Part model, mm, in its own coordinate system. A direction names the side the tool comes from. Give positions to 0.01 mm unless a question says otherwise; leave off trailing zeros. Write each loop counter-clockwise with the first axis right and the second up, starting at its lowest first coordinate (ties: lowest second). Pieces come first, ordered by that corner, then holes.
from build123d import *

# Parameters (mm, degrees)
SKETCH1_W               = 62
SKETCH1_H               = 48
BOSS_EXTRUDE1_DEPTH     = 5
SKETCH2_R               = 1.65
CUT_EXTRUDE2_DEPTH      = 5
SKETCH3_R               = 11
SKETCH3_R_2             = 1.65
BOSS_EXTRUDE2_DEPTH     = 2
SKETCH4_R               = 9.6
CUT_EXTRUDE4_DEPTH      = 5
SKETCH5_W               = 5
SKETCH5_H               = 35
BOSS_EXTRUDE3_DEPTH     = 25
CUT_EXTRUDE5_DEPTH      = 60.860253925
CUT_EXTRUDE5_DEPTH_BACK = 25
SKETCH6_R               = 1.15
SKETCH7_R               = 1.65
CUT_EXTRUDE6_DEPTH      = 5
SKETCH8_R               = 11
CUT_EXTRUDE7_DEPTH      = 65.536811201
SKETCH9_W               = 19
SKETCH9_H               = 60
BOSS_EXTRUDE4_DEPTH     = 3
SKETCH10_W              = 19
SKETCH10_H              = 55
BOSS_EXTRUDE5_DEPTH     = 3.7
SKETCH11_W              = 5
SKETCH11_H              = 48
BOSS_EXTRUDE6_DEPTH     = 25
BOSS_EXTRUDE7_DEPTH     = 3.7
SKETCH13_R              = 31
SKETCH13_R_2            = 28.5
BOSS_EXTRUDE8_DEPTH     = 25
SKETCH14_W              = 62
SKETCH14_H              = 5
BOSS_EXTRUDE9_DEPTH     = 10
SKETCH15_R              = 8
SKETCH15_R_2            = 7
BOSS_EXTRUDE10_DEPTH    = 7
CHAMFER1_SIZE           = 5
CUT_EXTRUDE8_DEPTH      = 109.894444303
CUT_EXTRUDE8_DEPTH_BACK = 109.894444303
SKETCH16_R              = 0.9
CHAMFER2_SIZE           = 5
SKETCH17_W              = 19
SKETCH17_H              = 60
CUT_EXTRUDE9_DEPTH      = 10
SKETCH18_W              = 30
SKETCH18_H              = 44.3
CUT_EXTRUDE10_DEPTH     = 10
CHAMFER3_SIZE           = 5


with BuildPart() as part:
    # Sketch1 → Boss-Extrude1 (new body)
    with BuildSketch(Plane.XY):
        Rectangle(SKETCH1_W, SKETCH1_H)
    extrude(amount=BOSS_EXTRUDE1_DEPTH)

    # Sketch2 → Cut-Extrude2 (cut)
    with BuildSketch(Plane.XY.offset(5)):
        with Locations((6, 7)):
            Circle(SKETCH2_R)
        with Locations((13, 0)):
            Circle(SKETCH2_R)
        with Locations((6, -7)):
            Circle(SKETCH2_R)
        with Locations((-1, 0)):
            Circle(SKETCH2_R)
    extrude(amount=-CUT_EXTRUDE2_DEPTH, mode=Mode.SUBTRACT)

    # Sketch3 → Boss-Extrude2 (add)
    with BuildSketch(Plane(origin=(0, 0, 0), x_dir=(-1, 0, 0), z_dir=(0, 0, -1))):
        with Locations(Location((-6, 0, 0), (0, 0, 180))):
            Circle(SKETCH3_R)
        with Locations(Location((1, 0, 0), (0, 0, 180))):
            Circle(SKETCH3_R_2, mode=Mode.SUBTRACT)
        with Locations(Location((-6, -7, 0), (0, 0, 180))):
            Circle(SKETCH3_R_2, mode=Mode.SUBTRACT)
        with Locations(Location((-13, 0, 0), (0, 0, 180))):
            Circle(SKETCH3_R_2, mode=Mode.SUBTRACT)
        with Locations(Location((-6, 7, 0), (0, 0, 180))):
            Circle(SKETCH3_R_2, mode=Mode.SUBTRACT)
    extrude(amount=BOSS_EXTRUDE2_DEPTH)

    # Sketch4 → Cut-Extrude4 (cut)
    with BuildSketch(Plane.XY.offset(5)):
        with Locations((6, 0)):
            Circle(SKETCH4_R)
    extrude(amount=-CUT_EXTRUDE4_DEPTH, mode=Mode.SUBTRACT)

    # Sketch5 → Boss-Extrude3 (add)
    with BuildSketch(Plane.XY.offset(5)):
        Polygon((8.15, -17.5), (8.15, -24), (31, -24), (31, -17.5), (26, -17.5), align=None)
        with Locations((28.5, 0)):
            Rectangle(SKETCH5_W, SKETCH5_H)
        Polygon((8.15, 17.5), (26, 17.5), (31, 17.5), (31, 24), (8.15, 24), align=None)
    extrude(amount=BOSS_EXTRUDE3_DEPTH)

    # Sketch6 → Cut-Extrude5 (cut, two sides: drawn at the far end of the back side and taken through both)
    with BuildSketch(Plane(origin=(0, -17.5, 0), x_dir=(1, 0, 0), z_dir=(0, 1, 0)).offset(-CUT_EXTRUDE5_DEPTH_BACK)):
        with Locations((20, -27.75)):
            Circle(SKETCH6_R)
        with Locations((20, -7.25)):
            Circle(SKETCH6_R)
        with Locations((-0.7, -7.25)):
            Circle(SKETCH6_R)
        with Locations((-0.7, -27.75)):
            Circle(SKETCH6_R)
    extrude(amount=CUT_EXTRUDE5_DEPTH + CUT_EXTRUDE5_DEPTH_BACK, mode=Mode.SUBTRACT)

    # Sketch7 → Cut-Extrude6 (cut)
    with BuildSketch(Plane(origin=(0, 24, 0), x_dir=(1, 0, 0), z_dir=(0, 1, 0))):
        with Locations((0.45, -7.25)):
            Circle(SKETCH7_R)
        with Locations(Location((20, -7.25, 0), (0, 0, 270))):
            Circle(SKETCH7_R)
        with Locations(Location((20, -27.75, 0), (0, 0, 270))):
            Circle(SKETCH7_R)
        with Locations((0.45, -27.75)):
            Circle(SKETCH7_R)
    cut_extrude6 = extrude(amount=-CUT_EXTRUDE6_DEPTH, mode=Mode.SUBTRACT)

    # Mirror1: Cut-Extrude6 across plane
    add(cut_extrude6.mirror(Plane.ZX), mode=Mode.SUBTRACT)

    # Sketch8 → Cut-Extrude7 (cut, through all)
    with BuildSketch(Plane(origin=(0, 24, 0), x_dir=(1, 0, 0), z_dir=(0, 1, 0))):
        with Locations((1.65, -17.5)):
            Circle(SKETCH8_R)
    extrude(amount=-CUT_EXTRUDE7_DEPTH, mode=Mode.SUBTRACT)

    # Sketch9 → Boss-Extrude4 (add)
    with BuildSketch(Plane(origin=(0, 24, 0), x_dir=(1, 0, 0), z_dir=(0, 1, 0))):
        with Locations((17.65, -60)):
            Rectangle(SKETCH9_W, SKETCH9_H)
    extrude(amount=-BOSS_EXTRUDE4_DEPTH)

    # Sketch10 → Boss-Extrude5 (add)
    with BuildSketch(Plane(origin=(0, 24, 0), x_dir=(1, 0, 0), z_dir=(0, 1, 0))):
        with Locations((17.65, -62.5)):
            Rectangle(SKETCH10_W, SKETCH10_H)
    extrude(amount=BOSS_EXTRUDE5_DEPTH)

    # Sketch11 → Boss-Extrude6 (add)
    with BuildSketch(Plane.XY.offset(5)):
        with Locations((-28.5, 0)):
            Rectangle(SKETCH11_W, SKETCH11_H)
    extrude(amount=BOSS_EXTRUDE6_DEPTH)

    # Sketch12 → Boss-Extrude7 (add)
    with BuildSketch(Plane.XZ.offset(24)):
        with BuildLine():
            Line((-31, 30), (31, 30))
            Line((31, 30), (31, 65))
            ThreePointArc((31, 65), (0, 96), (-31, 65))
            Line((-31, 65), (-31, 30))
        make_face()
    extrude(amount=-BOSS_EXTRUDE7_DEPTH)

    # Sketch13 → Boss-Extrude8 (add)
    with BuildSketch(Plane(origin=(0, -20.3, 0), x_dir=(1, 0, 0), z_dir=(0, 1, 0))):
        with Locations((0, -65)):
            Circle(SKETCH13_R)
        with Locations(Location((0, -65, 0), (0, 0, 270))):
            Circle(SKETCH13_R_2, mode=Mode.SUBTRACT)
    extrude(amount=BOSS_EXTRUDE8_DEPTH)

    # Sketch14 → Boss-Extrude9 (add)
    with BuildSketch(Plane(origin=(0, 24, 0), x_dir=(1, 0, 0), z_dir=(0, 1, 0))):
        with Locations((0, -2.5)):
            Rectangle(SKETCH14_W, SKETCH14_H)
    extrude(amount=BOSS_EXTRUDE9_DEPTH)

    # Sketch15 → Boss-Extrude10 (add)
    with BuildSketch(Plane(origin=(0, 34, 0), x_dir=(1, 0, 0), z_dir=(0, 1, 0))):
        with Locations(Location((0, -2.5, 0), (0, 0, 18.209956864))):
            Circle(SKETCH15_R)
        with Locations(Location((0, -2.5, 0), (0, 0, 159.075167572))):
            Circle(SKETCH15_R_2, mode=Mode.SUBTRACT)
    extrude(amount=BOSS_EXTRUDE10_DEPTH)

    # Chamfer1
    # the kernel refuses this chamfer: 5 mm, written as the material it adds along each edge
    with BuildSketch(Plane(origin=(0, 34, 2.5), x_dir=(0.34706049300703296, 0, -0.9378427449171398), z_dir=(0.9378427449171398, 0, 0.34706049300703296))) as chamfer1_piece_1_section:
        Polygon((8 + CHAMFER1_SIZE, 0), (8, CHAMFER1_SIZE), (8, 0), align=None)
    chamfer1_piece_1 = revolve(axis=Axis((0, 34, 2.5), (0, 1, 0)), revolution_arc=220.61525354, mode=Mode.PRIVATE)
    chamfer1_piece_1 = split(chamfer1_piece_1, bisect_by=Plane(origin=(-9.551791351, 35.668281916, 5), z_dir=(0, 0, -1)), keep=Keep.TOP, mode=Mode.PRIVATE)
    chamfer1_piece_1 = split(chamfer1_piece_1, bisect_by=Plane(origin=(-9.551791351, 35.668281916, 0), z_dir=(0, 0, 1)), keep=Keep.TOP, mode=Mode.PRIVATE)
    add(chamfer1_piece_1)
    with BuildSketch(Plane(origin=(0, 34, 2.5), x_dir=(-0.3470604930069759, 0, 0.9378427449171609), z_dir=(-0.9378427449171609, 0, -0.3470604930069759))) as chamfer1_piece_2_section:
        Polygon((8 + CHAMFER1_SIZE, 0), (8, CHAMFER1_SIZE), (8, 0), align=None)
    chamfer1_piece_2 = revolve(axis=Axis((0, 34, 2.5), (0, 1, 0)), revolution_arc=220.61525354, mode=Mode.PRIVATE)
    chamfer1_piece_2 = split(chamfer1_piece_2, bisect_by=Plane(origin=(9.551791351, 35.668281916, 5), z_dir=(0, 0, -1)), keep=Keep.TOP, mode=Mode.PRIVATE)
    chamfer1_piece_2 = split(chamfer1_piece_2, bisect_by=Plane(origin=(9.551791351, 35.668281916, 0), z_dir=(0, 0, 1)), keep=Keep.TOP, mode=Mode.PRIVATE)
    add(chamfer1_piece_2)

    # Sketch16 → Cut-Extrude8 (cut, two sides: drawn at the far end of the back side and taken through both)
    with BuildSketch(Plane(origin=(0, 0, 0), x_dir=(-1, 0, 0), z_dir=(0, 0, -1)).offset(-CUT_EXTRUDE8_DEPTH_BACK)):
        with Locations((0, 37.406113714)):
            Circle(SKETCH16_R)
    extrude(amount=CUT_EXTRUDE8_DEPTH + CUT_EXTRUDE8_DEPTH_BACK, mode=Mode.SUBTRACT)

    # Chamfer2
    # the kernel refuses this chamfer: 5 mm, written as the material it adds along each edge
    with BuildSketch(Plane(origin=(6.320066525, 34, 5), x_dir=(0, -0.9996219169112968, -0.027495876610586317), z_dir=(-1, 0, 0))) as chamfer2_piece_1_section:
        Polygon((CHAMFER2_SIZE * 0.999621916911, CHAMFER2_SIZE * 0.0274958766106), (-CHAMFER2_SIZE * 0.0274958766106, CHAMFER2_SIZE * 0.999621916911), (0, 0), align=None)
    chamfer2_piece_1 = extrude(amount=26.777823541, mode=Mode.PRIVATE)
    chamfer2_piece_1 = chamfer2_piece_1 & Plane(origin=(0, 31.52085101, 2.5), x_dir=(0.94991775959971, 0, -0.31249999999530786), z_dir=(0, -1, 0)) * Cylinder(8, 74, mode=Mode.PRIVATE)
    chamfer2_piece_1 = chamfer2_piece_1 - Plane(origin=(0, 31.52085101, 2.5), x_dir=(-0.9340497736136041, 0, -0.3571428571487537), z_dir=(0, -1, 0)) * Cylinder(7, 74, mode=Mode.PRIVATE)
    add(chamfer2_piece_1)
    with BuildSketch(Plane(origin=(20.457757017, 34, 5), x_dir=(0, -0.9996219169112968, -0.027495876610586317), z_dir=(-1, 0, 0))) as chamfer2_piece_2_section:
        Polygon((CHAMFER2_SIZE * 0.999621916911, CHAMFER2_SIZE * 0.0274958766106), (-CHAMFER2_SIZE * 0.0274958766106, CHAMFER2_SIZE * 0.999621916911), (0, 0), align=None)
    chamfer2_piece_2 = extrude(amount=26.777823541, mode=Mode.PRIVATE)
    chamfer2_piece_2 = chamfer2_piece_2 & Plane(origin=(0, 31.52085101, 2.5), x_dir=(0.94991775959971, 0, -0.31249999999530786), z_dir=(0, -1, 0)) * Cylinder(8, 74, mode=Mode.PRIVATE)
    chamfer2_piece_2 = chamfer2_piece_2 - Plane(origin=(0, 31.52085101, 2.5), x_dir=(-0.9340497736136041, 0, -0.3571428571487537), z_dir=(0, -1, 0)) * Cylinder(7, 74, mode=Mode.PRIVATE)
    add(chamfer2_piece_2)
    with BuildSketch(Plane(origin=(-6.320066525, 34, 0), x_dir=(0, -0.9996219169112968, 0.027495876610586372), z_dir=(1, 0, 0))) as chamfer2_piece_3_section:
        Polygon((CHAMFER2_SIZE * 0.999621916911, CHAMFER2_SIZE * 0.0274958766106), (-CHAMFER2_SIZE * 0.0274958766106, CHAMFER2_SIZE * 0.999621916911), (0, 0), align=None)
    chamfer2_piece_3 = extrude(amount=26.777823541, mode=Mode.PRIVATE)
    chamfer2_piece_3 = chamfer2_piece_3 & Plane(origin=(0, 31.52085101, 2.5), x_dir=(0.94991775959971, 0, -0.31249999999530786), z_dir=(0, -1, 0)) * Cylinder(8, 74, mode=Mode.PRIVATE)
    chamfer2_piece_3 = chamfer2_piece_3 - Plane(origin=(0, 31.52085101, 2.5), x_dir=(-0.9340497736136041, 0, -0.3571428571487537), z_dir=(0, -1, 0)) * Cylinder(7, 74, mode=Mode.PRIVATE)
    add(chamfer2_piece_3)
    with BuildSketch(Plane(origin=(-20.457757017, 34, 0), x_dir=(0, -0.9996219169112968, 0.027495876610586372), z_dir=(1, 0, 0))) as chamfer2_piece_4_section:
        Polygon((CHAMFER2_SIZE * 0.999621916911, CHAMFER2_SIZE * 0.0274958766106), (-CHAMFER2_SIZE * 0.0274958766106, CHAMFER2_SIZE * 0.999621916911), (0, 0), align=None)
    chamfer2_piece_4 = extrude(amount=26.777823541, mode=Mode.PRIVATE)
    chamfer2_piece_4 = chamfer2_piece_4 & Plane(origin=(0, 31.52085101, 2.5), x_dir=(0.94991775959971, 0, -0.31249999999530786), z_dir=(0, -1, 0)) * Cylinder(8, 74, mode=Mode.PRIVATE)
    chamfer2_piece_4 = chamfer2_piece_4 - Plane(origin=(0, 31.52085101, 2.5), x_dir=(-0.9340497736136041, 0, -0.3571428571487537), z_dir=(0, -1, 0)) * Cylinder(7, 74, mode=Mode.PRIVATE)
    add(chamfer2_piece_4)
    with BuildSketch(Plane(origin=(-31, -20.3, 30), x_dir=(0, -0.027495876610586317, 0.9996219169112968), z_dir=(1, 0, 0))) as chamfer2_piece_5:
        Polygon((CHAMFER2_SIZE * 0.999621916911, -CHAMFER2_SIZE * 0.0274958766106), (-CHAMFER2_SIZE * 0.0274958766106, -CHAMFER2_SIZE * 0.999621916911), (0, 0), align=None)
    extrude(amount=5)

    # Sketch17 → Cut-Extrude9 (cut)
    with BuildSketch(Plane(origin=(0, 27.7, 0), x_dir=(1, 0, 0), z_dir=(0, 1, 0))):
        with Locations((17.65, -60)):
            Rectangle(SKETCH17_W, SKETCH17_H)
    extrude(amount=-CUT_EXTRUDE9_DEPTH, mode=Mode.SUBTRACT)

    # Sketch18 → Cut-Extrude10 (cut)
    with BuildSketch(Plane.ZY.offset(31)):
        with Locations((20, 1.85)):
            Rectangle(SKETCH18_W, SKETCH18_H)
    extrude(amount=-CUT_EXTRUDE10_DEPTH, mode=Mode.SUBTRACT)

    # Chamfer3
    chamfer3_edges = [part.edges().sort_by_distance(p)[0] for p in [
        (-28.5, -20.3, 5),
    ]]
    chamfer(chamfer3_edges, length=CHAMFER3_SIZE)


solid = part.part
1) Saw through at A-A (z = 2.5). Write the cut outline in (x, y), and give its area (3 significant figures).
Check result:
outline: (-31, -24) - (31, -24) - (31, 34) - (13, 34) - (8, 39) - (8, 41) - (7, 41) - (7, 34) - (-7, 34) - (-7, 41) - (-8, 41) - (-8, 39) - (-13, 34) - (-31, 34) - close; hole circle Ø19.2 at (6, 0)
area: 3,350 mm2
2) Drill centre lines: L1, parallel to X at y = -21.15, z = 27.75; L2, parallel to Z at x = 17.5, y = -17; L3, parallel to X at y = 22, z = 7. Where is each one in solid material? Low to high.
Check result:
L1: x = -31 to -26, 8.15 to 18.35, 21.65 to 31
L2: z = 0 to 5, 39.41 to 42.51, 87.49 to 90.59
L3: x = 8.15 to 18.37, 21.63 to 31
3) Flat gauge pins, fed straight in: P1, Ø10, axis at x = -19, y = 0.5, coming from the -Z side; P2, Ø2.5, axis at x = 20, z = 27.75, coming from the +Y side; P3, Ø19.5, axis at x = 17, z = 18, coming from the +Y side; P4, Ø1, axis at x = -2, z = 12.5, coming from the +Y side. Where does each tip first touch, or does it go through?
Check result:
P1: stops at z = 0
P2: stops at y = 19
P3: stops at y = 24
P4: passes through
4) 3-axis set-ups, long thin cutter, end or side, ignore diameter. For faces 1 (the cylindrical face through (-6.72, -9.851, 95.263)), 2 (the flat face through (19, 24, 17)), 3 (the flat face through (18.9, -19, 28.5)): which of +Z, -Z, +X, -X, +Y, -Y reach the whole face in a straight line?
Check result:
face 1: +Y
face 2: +Z, +X, -X, +Y
face 3: -Y
5) Saw through at C-C (y = 15.5). Write the cut outline in (x, z), and give its area (3 significant figures).
Check result:
outline: (-31, 0) - (31, 0) - (31, 30) - (26, 30) - (26, 5) - (-31, 5) - close
area: 435 mm2
6) Saw through at B-B (y = 7). Write the cut outline in (x, z), and give its area (3 significant figures).
Check result:
outline: (-31, 0) - (-2.49, 0) - (-2.49, -2) - (4.35, -2) - (4.35, 0) - (-0.57, 0) - (-0.57, 5) - (-31, 5) - close; (7.65, -2) - (14.49, -2) - (14.49, 0) - (31, 0) - (31, 30) - (26, 30) - (26, 5) - (12.57, 5) - (12.57, 0) - (7.65, 0) - close
area: 397 mm2
7) Saw through at D-D (z = 50). Write the cut outline in (x, y).
Check result:
outline: (-31, -24) - (31, -24) - (31, -20.3) - (27.13, -20.3) - (27.13, 4.7) - (24.23, 4.7) - (24.23, -20.3) - (-24.23, -20.3) - (-24.23, 4.7) - (-27.13, 4.7) - (-27.13, -20.3) - (-31, -20.3) - close
8) Mould opens along Z. For faces 4 (the cylindrical face through (4.69, -6, -0.99)), 5 (the flat face through (8.15, -21, 7)) say: +Z half, -Z half, draft (parallel to the pull), parting line (faces both ways), or undercut.
Check result:
face 4: draft
face 5: undercut
